The listing builds one solid part. Answer for the finished solid, in the listing's coordinates (mm). A direction names the side the tool comes from. Give positions to 0.01 mm unless a question says otherwise; leave off trailing zeros. Loops run counter-clockwise (first coordinate to the right, second up) from the corner with the lowest first, then second, coordinate; pieces in that order, holes last. Notation, with made-up numbers: M -35,86.25 L -26,86.25 A14 ccw -26,108.25 Z; hole C 12,61.5 d4. An arc over 180 degrees is marked long. Use one line per item in the form item = value. Start each with the question number.
1. The part is cut by section C-C (z = 190.5). Write down the section's boundary in (x, y), and give its area (3 significant figures).
2. Straight lines are drawn through the part: line 1 (Z direction, x = 5, y = 11); line 2 (Z direction, x = 4.5, y = 7.25); line 3 (X direction, y = 5, z = 160). For each, find the intervals that lie inside material, in ascending order. Write a range as from..to.
3. The mould has two halves that part along X. Classify faces 1 (the face through (0, 8, 158)), 2 (the face through (7.48, 7.6, 9.67)), 3 (the face through (5, 8, 320)), 4 (the face through (8.479, 12.056, 157.76)): released by +X, released by -X, zero draft, split by the parting line, or undercut.
4. Each of these flat-tipped pins is pushed along its axis until it touches: pin 1 Ø5 at (y, z) = (13.5, 136.5) entering from +X (3 decimals); pin 2 Ø4.5 at (x, z) = (5, 160) entering from -Y. Where does it stop, or does it pass through?
5. For faces 5 (the face through (10, 4, 158)), 6 (the face through (4.04, 7.6, 312.31)), determine the directions among +Z, -Z, +X, -X, +Y, -Y from which every point of the face is accessible in a straight line to the end or side of a thin tool.
6. The part is cut by section A-A (y = 2.75). Write down the section's boundary in (x, z), and give its area (3 significant figures).
7. The part is cut by section B-B (x = 5). Write down the section's boundary in (y, z).
from build123d import *

# Parameters (mm, degrees)
SKETCH_1_W             = 10
SKETCH_1_H             = 16
EXTRUDE_1_DEPTH        = 320
HOLE_WIZARD_M6_1_D     = 5
HOLE_WIZARD_M6_1_DEPTH = 15
HOLE_WIZARD_M6_1_TIP   = 1.502151548
CHAMFER_1_SIZE         = 8
CHAMFER_1_SIZE2        = 3


with BuildPart() as part:
    # 草图1 → 凸台-拉伸1 (new body)
    with BuildSketch(Plane.XY):
        with Locations((5, 8)):
            Rectangle(SKETCH_1_W, SKETCH_1_H)
    extrude(amount=EXTRUDE_1_DEPTH)

    # M6 螺纹孔1
    with Locations(Plane(origin=(5, 0, 310), x_dir=(0, 0, -1), z_dir=(0, -1, 0))):
        with Locations((0, 0), (150, 0), (300, 0)):
            Hole(HOLE_WIZARD_M6_1_D / 2, depth=HOLE_WIZARD_M6_1_DEPTH)
            with Locations((0, 0, -(HOLE_WIZARD_M6_1_DEPTH + HOLE_WIZARD_M6_1_TIP / 2))):  # 118° drill point
                Cone(0, HOLE_WIZARD_M6_1_D / 2, HOLE_WIZARD_M6_1_TIP, mode=Mode.SUBTRACT)

    # 倒角1
    chamfer_1_edges = [part.edges().sort_by_distance(p)[0] for p in [
        (10, 16, 160),
    ]]
    chamfer_1_side = [part.faces().sort_by_distance(p)[0] for p in [
        (10, 8, 160),
    ]]
    chamfer(chamfer_1_edges, length=CHAMFER_1_SIZE, length2=CHAMFER_1_SIZE2, reference=chamfer_1_side[0])


solid = part.part
Derived:
q1.outline = M 0,0 L 10,0 L 10,8 L 7,16 L 0,16 Z
q1.area = 148 mm2
q2.line_1 = 0..7.5, 12.5..157.5, 162.5..307.5, 312.5..320
q2.line_2 = 0..7.55, 12.45..157.55, 162.45..307.55, 312.45..320
q2.line_3 = 0..2.5, 7.5..10
q3.face_1 = released by -X
q3.face_2 = undercut
q3.face_3 = zero draft
q3.face_4 = released by +X
q4.pin_1 = 8.875
q4.pin_2 = 15.15
q5.face_5 = +Z, -Z, +X, +Y, -Y
q5.face_6 = -Y
q6.outline = M 0,0 L 10,0 L 10,320 L 0,320 Z; hole C 5,10 d5; hole C 5,160 d5; hole C 5,310 d5
q6.area = 3,140 mm2
q7.outline = M 0,0 L 16,0 L 16,9.16 L 15,7.5 L 0,7.5 Z; M 0,12.5 L 15,12.5 L 16,10.84 L 16,159.16 L 15,157.5 L 0,157.5 Z; M 0,162.5 L 15,162.5 L 16,160.84 L 16,309.16 L 15,307.5 L 0,307.5 Z; M 0,312.5 L 15,312.5 L 16,310.84 L 16,320 L 0,320 Z
